For this review, take the finished solid that the model builds, in its own axes (mm). A direction names the side the tool comes from. Give positions to 0.01 mm unless a question says otherwise; leave off trailing zeros. Write each loop counter-clockwise with the first axis right and the second up, starting at its lowest first coordinate (ties: lowest second). Pieces come first, ordered by that corner, then holes. Notation, with made-up numbers: (84, 61) -> (121, 61) arc R19 ccw to (121, 81) -> close; hole circle Ø3 at (62.25, 0.25). An arc over 180 degrees is marked (long way). Write item = value, one per line.
```python
from build123d import *

# Parameters (mm, degrees)
SKETCH1_W           = 99
SKETCH1_H           = 194
BOSS_EXTRUDE1_DEPTH = 3
SKETCH2_W           = 43
SKETCH2_H           = 7
CUT_EXTRUDE1_DEPTH  = 4
FILLET1_R           = 1
SKETCH3_R           = 8.5
SKETCH3_R_2         = 3.1
CUT_EXTRUDE2_DEPTH  = 4
SKETCH4_W           = 45
SKETCH4_H           = 26
CUT_EXTRUDE3_DEPTH  = 1.5
FILLET2_R           = 3
SKETCH5_R           = 2.75
CUT_EXTRUDE4_DEPTH  = 4


with BuildPart() as part:
    # Sketch1 → Boss-Extrude1 (new body)
    with BuildSketch(Plane.ZY.offset(74.98828393)):
        with Locations((-16.230657269, 7.5)):
            Rectangle(SKETCH1_W, SKETCH1_H)
    extrude(amount=BOSS_EXTRUDE1_DEPTH)

    # Sketch2 → Cut-Extrude1 (cut, through all)
    with BuildSketch(Plane.ZY.offset(77.98828393)):
        with Locations((-16.230657269, 73.75)):
            Rectangle(SKETCH2_W, SKETCH2_H)
        with Locations((-16.230657269, 62.15)):
            Rectangle(SKETCH2_W, SKETCH2_H)
        with Locations((-16.230657269, 50.55)):
            Rectangle(SKETCH2_W, SKETCH2_H)
        with Locations((-16.230657269, 38.95)):
            Rectangle(SKETCH2_W, SKETCH2_H)
        with Locations((-16.230657269, 27.35)):
            Rectangle(SKETCH2_W, SKETCH2_H)
        with Locations((-16.230657269, 15.75)):
            Rectangle(SKETCH2_W, SKETCH2_H)
        with Locations((-16.230657269, 4.15)):
            Rectangle(SKETCH2_W, SKETCH2_H)
    extrude(amount=-CUT_EXTRUDE1_DEPTH, mode=Mode.SUBTRACT)

    # Fillet1
    fillet1_edges = [part.edges().sort_by_distance(p)[0] for p in [
        (-76.48828393, 77.25, 5.269342731),
        (-76.48828393, 70.25, 5.269342731),
        (-76.48828393, 70.25, -37.730657269),
        (-76.48828393, 77.25, -37.730657269),
        (-76.48828393, 65.65, 5.269342731),
        (-76.48828393, 58.65, 5.269342731),
        (-76.48828393, 58.65, -37.730657269),
        (-76.48828393, 65.65, -37.730657269),
        (-76.48828393, 54.05, 5.269342731),
        (-76.48828393, 47.05, 5.269342731),
        (-76.48828393, 47.05, -37.730657269),
        (-76.48828393, 54.05, -37.730657269),
        (-76.48828393, 42.45, 5.269342731),
        (-76.48828393, 35.45, 5.269342731),
        (-76.48828393, 35.45, -37.730657269),
        (-76.48828393, 42.45, -37.730657269),
        (-76.48828393, 30.85, 5.269342731),
        (-76.48828393, 23.85, 5.269342731),
        (-76.48828393, 23.85, -37.730657269),
        (-76.48828393, 30.85, -37.730657269),
        (-76.48828393, 19.25, 5.269342731),
        (-76.48828393, 12.25, 5.269342731),
        (-76.48828393, 12.25, -37.730657269),
        (-76.48828393, 19.25, -37.730657269),
        (-76.48828393, 7.65, 5.269342731),
        (-76.48828393, 0.65, 5.269342731),
        (-76.48828393, 0.65, -37.730657269),
        (-76.48828393, 7.65, -37.730657269),
    ]]
    fillet(fillet1_edges, radius=FILLET1_R)

    # Sketch3 → Cut-Extrude2 (cut, through all)
    with BuildSketch(Plane.ZY.offset(77.98828393)):
        with Locations((-16.230657269, -50)):
            Circle(SKETCH3_R)
        with Locations((-41.230657269, -50)):
            Circle(SKETCH3_R_2)
    extrude(amount=-CUT_EXTRUDE2_DEPTH, mode=Mode.SUBTRACT)

    # Sketch4 → Cut-Extrude3 (cut)
    with BuildSketch(Plane(origin=(-74.98828393, 0, 0), x_dir=(0, 0, -1), z_dir=(1, 0, 0))):
        with Locations((25.730657269, -50)):
            Rectangle(SKETCH4_W, SKETCH4_H)
    extrude(amount=-CUT_EXTRUDE3_DEPTH, mode=Mode.SUBTRACT)

    # Fillet2
    fillet2_edges = [part.edges().sort_by_distance(p)[0] for p in [
        (-75.73828393, -37, -48.230657269),
        (-75.73828393, -63, -48.230657269),
        (-75.73828393, -63, -3.230657269),
        (-75.73828393, -37, -3.230657269),
    ]]
    fillet(fillet2_edges, radius=FILLET2_R)

    # Sketch5 → Cut-Extrude4 (cut, through all)
    with BuildSketch(Plane.ZY.offset(77.98828393)):
        with Locations((-61.230657269, 100)):
            Circle(SKETCH5_R)
        with Locations((28.769342731, 100)):
            Circle(SKETCH5_R)
        with Locations((-61.230657269, -15)):
            Circle(SKETCH5_R)
        with Locations((-61.230657269, -85)):
            Circle(SKETCH5_R)
        with Locations((28.769342731, -85)):
            Circle(SKETCH5_R)
        with Locations((28.769342731, -15)):
            Circle(SKETCH5_R)
        with Locations((-16.230657269, 100)):
            Circle(SKETCH5_R)
        with Locations((-16.230657269, -85)):
            Circle(SKETCH5_R)
    extrude(amount=-CUT_EXTRUDE4_DEPTH, mode=Mode.SUBTRACT)


solid = part.part
```
(1) Take a section at D-D (z = -40.5). Write out the cut boundary in (x, y).
Answers below:
outline = (-77.99, -89.5) -> (-74.99, -89.5) -> (-74.99, -63) -> (-76.49, -63) -> (-76.49, -53.01) -> (-77.99, -53.01) -> close; (-77.99, -46.99) -> (-76.49, -46.99) -> (-76.49, -37) -> (-74.99, -37) -> (-74.99, 104.5) -> (-77.99, 104.5) -> close
(2) Take a section at B-B (y = -50). Write out the cut boundary in (x, z).
Answers below:
outline = (-77.99, -65.73) -> (-74.99, -65.73) -> (-74.99, -48.23) -> (-76.49, -48.23) -> (-76.49, -44.33) -> (-77.99, -44.33) -> close; (-77.99, -38.13) -> (-76.49, -38.13) -> (-76.49, -24.73) -> (-77.99, -24.73) -> close; (-77.99, -7.73) -> (-76.49, -7.73) -> (-76.49, -3.23) -> (-74.99, -3.23) -> (-74.99, 33.27) -> (-77.99, 33.27) -> close
(3) Take a section at C-C (y = 100). Write out the cut boundary in (x, z), plus the area to 4 significant figures.
Answers below:
outline = (-77.99, -65.73) -> (-74.99, -65.73) -> (-74.99, -63.98) -> (-77.99, -63.98) -> close; (-77.99, -58.48) -> (-74.99, -58.48) -> (-74.99, -18.98) -> (-77.99, -18.98) -> close; (-77.99, -13.48) -> (-74.99, -13.48) -> (-74.99, 26.02) -> (-77.99, 26.02) -> close; (-77.99, 31.52) -> (-74.99, 31.52) -> (-74.99, 33.27) -> (-77.99, 33.27) -> close
area = 247.5 mm^2
(4) Tool access review of faces 4 (the face through (-76.51, -14.88, -63.98)), 5 (the face through (-76.488, -50, -25)): name each direction out of +Z, -Z, +X, -X, +Y, -Y from which nothing blocks a thin tool from reaching the whole face with its end or side.
Answers below:
face_4 = +X, -X
face_5 = +X
(5) Take a section at A-A (y = 50). Write out the cut boundary in (x, z), plus the area to 3 significant figures.
Answers below:
outline = (-77.99, -65.73) -> (-74.99, -65.73) -> (-74.99, -37.73) -> (-77.99, -37.73) -> close; (-77.99, 5.27) -> (-74.99, 5.27) -> (-74.99, 33.27) -> (-77.99, 33.27) -> close
area = 168 mm^2
(6) To check wall thickness, follow probe 1 along Z at (x, y) = (-76.35, 50); probe 2 along Z at (x, y) = (-77.25, -16); probe 3 along X at (y, z) = (-50, -31). State the ranges of each line that lie inside material, in increasing order.
Answers below:
probe_1 = -65.73 to -37.73, 5.27 to 33.27
probe_2 = -65.73 to -63.79, -58.67 to 26.21, 31.33 to 33.27
probe_3 = -77.99 to -76.49
(7) For pin 1 (5 mm diameter, centred on y = -50, z = -41.23, fed in from -X) (3 decimals), flat-tipped, find the tip position at first contact; note if it passes through.
Answers below:
pin_1 = through
(8) The part is to be moulded in two halves that separate along Z. For faces 1 (the face through (-76.509, 97.315, -16.827)), 2 (the face through (-76.5, -84.2, 31.4)), 3 (the face through (-77.988, 9, -17)), say which applies: released by +Z, released by -Z, zero draft, split by the parting line, or undercut.
Answers below:
face_1 = undercut
face_2 = undercut
face_3 = zero draft
